CAD build for the part. Positions are in the model's coordinates, mm. A direction names the side the tool comes from. Coordinates: 2 decimals unless noted, no trailing zeros. Loops run counter-clockwise (first coordinate to the right, second up) from the corner with the lowest first, then second, coordinate; pieces in that order, holes last.
1) Two-plate mould, pull along Y, no slides. Class faces 4 (the flat face through (-321.613, 16, 1167)), 5 (the cylindrical face through (-349.753, 38.623, 1161.91)), 6 (the flat face through (-400.053, 17, 1168)), 7 (the cylindrical face through (-399.45, 55.11, 1155.46)): +Y half, -Y half, draft (parallel to the pull), parting line (faces both ways), or undercut.
2) Wall check: line 1 along X through (y, z) = (27, 1168.5); line 2 along X through (y, z) = (43, 1172.5); line 3 along Y through (x, z) = (-332, 1161.5). Give the ranges that are in metal, low to high.
3) Which spindle directions (+Z, -Z, +X, -X, +Y, -Y) get a long thin tool onto all of the face, cutting with end or side? Do faces 1 (the cylindrical face through (-375.249, 37.132, 1163.544)), 2 (the flat face through (-348.613, 48, 1160)), 3 (the flat face through (-362, -24.323, 1167)). Say none if no direction does.
4) Pin check, flat tips, straight feed: pin 1 Ø9 at (x, z) = (-363.5, 1155.5) entering from +Y; pin 2 Ø3 at (x, y) = (-384.5, 13.5) entering from +Z. Stop position of each tip, or through.
5) Saw through at B-B, the plane y = -14. Write the cut outline in (x, z), and give its area (3 significant figures).
```python
from build123d import *

# Parameters (mm, degrees)
BOSS_EXTRUDE2_DEPTH      = 10
BOSS_EXTRUDE2_DEPTH_BACK = 51
SHELL2_T                 = -2
CUT_EXTRUDE2_DEPTH       = 81.44
SKETCH4_R                = 5.05
CUT_EXTRUDE3_DEPTH       = 62.0000001


with BuildPart() as part:
    # Sketch1 → Boss-Extrude2 (new body, two sides)
    with BuildSketch(Plane(origin=(0, 0, 1146.708434145), x_dir=(-1, 0, 0), z_dir=(0, 0, -1))) as boss_extrude2_sk:
        with BuildLine():
            Line((398.052845122, -24.322837047), (325.612845122, -24.322837047))
            ThreePointArc((325.612845122, -24.322837047), (322.784417997, -23.151264171), (321.612845122, -20.322837047))
            Line((321.612845122, -20.322837047), (321.612845122, 53.677162953))
            ThreePointArc((321.612845122, 53.677162953), (322.784417997, 56.505590078), (325.612845122, 57.677162953))
            Line((325.612845122, 57.677162953), (344.612845122, 57.677162953))
            ThreePointArc((344.612845122, 57.677162953), (347.441272247, 56.505590078), (348.612845122, 53.677162953))
            Line((348.612845122, 53.677162953), (348.612845122, 41.420568524))
            ThreePointArc((348.612845122, 41.420568524), (349.784417997, 38.5921414), (352.612845122, 37.420568524))
            Line((352.612845122, 37.420568524), (371.052845122, 37.420568524))
            ThreePointArc((371.052845122, 37.420568524), (373.881272247, 38.5921414), (375.052845122, 41.420568524))
            Line((375.052845122, 41.420568524), (375.052845122, 53.677162953))
            ThreePointArc((375.052845122, 53.677162953), (376.224417997, 56.505590078), (379.052845122, 57.677162953))
            Line((379.052845122, 57.677162953), (398.052845122, 57.677162953))
            ThreePointArc((398.052845122, 57.677162953), (400.881272247, 56.505590078), (402.052845122, 53.677162953))
            Line((402.052845122, 53.677162953), (402.052845122, -20.322837047))
            ThreePointArc((402.052845122, -20.322837047), (400.881272247, -23.151264171), (398.052845122, -24.322837047))
        make_face()
    extrude(amount=BOSS_EXTRUDE2_DEPTH)
    extrude(boss_extrude2_sk.sketch, amount=-BOSS_EXTRUDE2_DEPTH_BACK)

    # Shell2
    shell2_openings = [part.faces().sort_by_distance(p)[0] for p in [
        (-361.832845122, 32.113014346, 1197.708434145),
    ]]
    offset(amount=SHELL2_T, openings=shell2_openings, kind=Kind.INTERSECTION)

    # Sketch2 → Cut-Extrude2 (cut, through all)
    with BuildSketch(Plane(origin=(-321.612845122, 0, 0), x_dir=(0, 0, -1), z_dir=(1, 0, 0))):
        with BuildLine():
            Line((-1197.708434145, 4.331235789), (-1202.700494478, 4.331235789))
            Line((-1202.700494478, 4.331235789), (-1202.700494478, 60.889226386))
            Line((-1202.700494478, 60.889226386), (-1167.208434145, 60.889226386))
            Line((-1167.208434145, 60.889226386), (-1167.208434145, 57.677162953))
            add(Edge.make_bspline(
                [(-1197.708434145, 4.331235789), (-1197.068834598, 37.525012085), (-1167.208434145, 57.677162953)],
                knots=[0, 0, 0, 1, 1, 1], degree=2))
        make_face()
    extrude(amount=-CUT_EXTRUDE2_DEPTH, mode=Mode.SUBTRACT)

    # Sketch4 → Cut-Extrude3 (cut, through all)
    with BuildSketch(Plane(origin=(0, 0, 1136.708434145), x_dir=(-1, 0, 0), z_dir=(0, 0, -1))):
        with Locations((335.112845122, 47.548865739)):
            Circle(SKETCH4_R)
    extrude(amount=-CUT_EXTRUDE3_DEPTH, mode=Mode.SUBTRACT)


solid = part.part
```
Data:
1. face 4: draft
1. face 5: +Y half
1. face 6: undercut
1. face 7: undercut
2. line 1: x = -402.05 to -400.05, -323.61 to -321.61
2. line 2: x = -402.05 to -400.05, -377.05 to -375.05, -348.61 to -346.61, -323.61 to -321.61
2. line 3: y = -24.32 to -22.32, 55.68 to 57.68
3. face 1: +Z
3. face 2: +Z, -Z, +Y
3. face 3: +Z, -Z, +X, -X, -Y
4. pin 1: stops at y = 37.42
4. pin 2: stops at z = 1138.71
5. outline: (-402.05, 1136.71) - (-321.61, 1136.71) - (-321.61, 1197.71) - (-323.61, 1197.71) - (-323.61, 1138.71) - (-400.05, 1138.71) - (-400.05, 1197.71) - (-402.05, 1197.71) - close
5. area: 397 mm2
